Build history of the part. All positions in model axes, mm. Face numbers are marked on the shaded views. A direction names the side the tool comes from. Give positions to 0.01 mm unless a question says otherwise; leave off trailing zeros. Order: outer loops, then holes, each group sorted by start corner. A loop starts at its lowest first (then second) coordinate and runs counter-clockwise, first axis right, second up. Notation, with made-up numbers: (-12, 57) -> (-3, 57) arc R29 ccw to (-3, 96) -> close; hole circle Ø6 at (-16.5, 55.25). An arc over 180 degrees is marked (long way). One line per item, written item: value. Start each with the question number.
(1) Saw through at A-A on z = 15.5. Give the cut face in (x, y), plus the area to 3 significant figures.
(2) Pin check, flat tips, straight feed: pin 1 (12.5 mm diameter, centred on x = -2, z = -5, fed in from +Y); pin 2 (0.7 mm diameter, centred on x = -16, z = -16, fed in from +Y); pin 3 (1.2 mm diameter, centred on x = 15, z = -15, fed in from +Y); pin 4 (8 mm diameter, centred on x = -9.5, z = 6.5, fed in from +Y). Stop position of each tip, or through.
(3) Saw through at D-D on z = -9. Give the cut face in (x, y).
(4) Saw through at C-C on y = 54.5. Give the cut face in (x, z).
(5) Which spindle directions (+Z, -Z, +X, -X, +Y, -Y) get a long thin tool onto all of the face, cutting with end or side? Do the marked faces 1 and 2. Say none if no direction does.
(6) Probe line 1 (X direction, y = 45.5, z = 15.5); line 2 (X direction, y = 46, z = -15). List the from-to ranges inside material, lowest first.
(7) Saw through at B-B on x = 0. Give the cut face in (y, z).
Autodesk Inventor part; units mm, degrees
ref_plane "YZ Plane" through (0, 0, 0) normal (1, 0, 0) x (0, 1, 0)
ref_plane "XZ Plane" through (0, 0, 0) normal (0, 1, 0) x (-1, 0, 0)
ref_plane "XY Plane" through (0, 0, 0) normal (0, 0, 1) x (1, 0, 0)
sketch "Sketch1" plane through (0, 0, 0) normal (0, 1, 0) x (-1, 0, 0)
  line L0 (-21.15, -21.15) -> (21.15, -21.15)
  line L1 (21.15, -21.15) -> (21.15, 21.15)
  line L2 (21.15, 21.15) -> (-21.15, 21.15)
  line L3 (-21.15, 21.15) -> (-21.15, -21.15)
  line L4 (-21.15, -21.15) -> (21.15, 21.15) construction
  line L5 (21.15, -21.15) -> (-21.15, 21.15) construction
  point P0 (0, 0)
  dimension "d0" = 42.3
  dimension "d1" = 42.3
extrude "Extrusion1" add sketch "Sketch1" along normal blind 48
sketch "Sketch2" plane through (0, 48, 0) normal (0, 1, 0) x (1, 0, 0)
  circle A0 centre (0, 0) radius 11
  dimension "d4" = 22
extrude "Extrusion2" add sketch "Sketch2" along normal blind 2
sketch "Sketch3" plane through (0, 50, 0) normal (0, 1, 0) x (1, 0, 0)
  circle A0 centre (0, 0) radius 11
  circle A1 centre (0, 0) radius 2.5
  dimension "d7" = 5
extrude "Extrusion3" add sketch "Sketch3" along normal blind 22 contours A1
sketch "Sketch4" plane through (0, 48, 0) normal (0, 1, 0) x (1, 0, 0)
  circle A0 centre (0, 0) radius 11
  line L0 (-15.5, 15.5) -> (15.5, 15.5) construction
  line L1 (15.5, 15.5) -> (15.5, -15.5) construction
  line L2 (15.5, -15.5) -> (-15.5, -15.5) construction
  line L3 (-15.5, -15.5) -> (-15.5, 15.5) construction
  dimension "d10" = 31
  dimension "d11" = 31
  dimension "d12" = 15.5
  dimension "d13" = 15.5
hole "Hole1" at (-15.5, 48, -15.5) at (15.5, 48, -15.5) at (15.5, 48, 15.5) at (-15.5, 48, 15.5) direction (0, -1, 0) diameter 2.459 depth 4.5
sketch "Sketch5" plane through (21.15, 0, 21.15) normal (1, 0, 0) x (0, 0, -1)
  line L0 (0, 0) -> (42.3, 0)
  line L1 (42.3, 0) -> (42.3, 48)
  line L2 (0, 48) -> (42.3, 48)
  line L3 (0, 0) -> (0, 48)
  line L4 (26.15, 0) -> (26.15, 10)
  line L5 (26.15, 10) -> (16.15, 10)
  line L6 (16.15, 10) -> (16.15, 0)
  line L7 (16.15, 10) -> (26.15, 0)
  line L8 (26.15, 10) -> (16.15, 0)
  line L9 (18.65, 2.5) -> (23.65, 2.5)
  line L10 (23.65, 2.5) -> (23.65, 7.5)
  line L11 (23.65, 7.5) -> (18.65, 7.5)
  line L12 (18.65, 7.5) -> (18.65, 2.5)
  line L13 (18.65, 2.5) -> (23.65, 7.5) construction
  line L14 (23.65, 2.5) -> (18.65, 7.5) construction
  point P0 (21.15, 0)
  point P1 (21.15, 5)
  dimension "d23" = 16.15
  dimension "d24" = 16.15
  dimension "d26" = 10
  dimension "d27" = 10
  dimension "d28" = 5
  dimension "d29" = 5
properties part number "NEMA_17" material "Steel, Carbon"
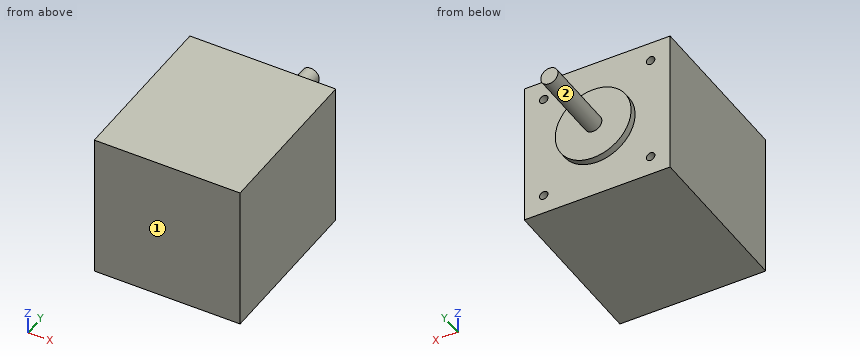
Results below:
1. outline: (-21.15, 0) -> (21.15, 0) -> (21.15, 48) -> (16.73, 48) -> (16.73, 43.5) -> (14.27, 43.5) -> (14.27, 48) -> (-14.27, 48) -> (-14.27, 43.5) -> (-16.73, 43.5) -> (-16.73, 48) -> (-21.15, 48) -> close
1. area: 2,010 mm²
2. pin 1: stops at y = 72
2. pin 2: stops at y = 43.5
2. pin 3: stops at y = 48
2. pin 4: stops at y = 50
3. outline: (-21.15, 0) -> (21.15, 0) -> (21.15, 48) -> (6.32, 48) -> (6.32, 50) -> (-6.32, 50) -> (-6.32, 48) -> (-21.15, 48) -> close
4. outline: circle Ø5 at (0, 0)
5. face 1: +Z, -Z, +X, -X, -Y
5. face 2: +Y
6. line 1: x = -21.15 to -16.73, -14.27 to 14.27, 16.73 to 21.15
6. line 2: x = -21.15 to -16.62, -14.38 to 14.38, 16.62 to 21.15
7. outline: (0, -21.15) -> (48, -21.15) -> (48, -11) -> (50, -11) -> (50, -2.5) -> (72, -2.5) -> (72, 2.5) -> (50, 2.5) -> (50, 11) -> (48, 11) -> (48, 21.15) -> (0, 21.15) -> close
